Verification items for the finished model (mm, model axes). A direction names the side the tool comes from. Give positions to 0.01 mm unless a question says otherwise; leave off trailing zeros. Order: outer loops, then holes, each group sorted by start corner. A loop starts at its lowest first (then second) coordinate and runs counter-clockwise, first axis right, second up.
(1) Scan lines: L1, parallel to X at y = 32, z = 26.7; L2, parallel to Y at x = 66.5, z = 3.4; L3, parallel to X at y = -24, z = 17.5. Record each from-to range of solid material in increasing order.
(2) Sectioned sample at B-B on y = 4. Record the cut outline in (x, z), plus the area to 3 significant figures.
(3) Gauge pin test, flat ends, axial feed: pin 1 (2.5 mm diameter, centred on y = -32.5, z = 28, fed in from +X); pin 2 (1.5 mm diameter, centred on y = -30.5, z = 1, fed in from -X); pin 3 (12 mm diameter, centred on x = 47, z = 1, fed in from -Y); pin 4 (1.5 mm diameter, centred on x = 37.5, y = -25, fed in from +Z). Record the tip position at first contact, or that the pin passes through.
(4) Sectioned sample at A-A on x = -55.5. Record the cut outline in (y, z), plus the area to 3 significant figures.
(5) Access from +Z, -Z, +X, -X, +Y, -Y to the whole of each face (thin tool, end or side, straight path). Record for faces 1 (the face through (59.5, 32, 28)), 2 (the face through (69.5, 32, 28)), 3 (the face through (-59.5, -32, -3)).
(6) Mould release check, pull along Y, two halves, no side actions. Record for faces 4 (the face through (-69.5, -32, 28)), 5 (the face through (66.24, -20.517, 2.465)), 6 (the face through (60.93, 38, -2.97)), 7 (the face through (-68.07, -38, -2.97)): pulls with the +Y half, pulls with the -Y half, needs draft (parallel to the pull), parting line crosses it, or undercut.
```python
from build123d import *

# Parameters (mm, degrees)
F0_W      = 149
F0_H      = 59
F0_W_2    = 145
F0_H_2    = 55
F1_DEPTH  = 30
F2_W      = 149
F2_H      = 59
F2_W_2    = 145
F2_H_2    = 55
F3_DEPTH  = 5
F4_R      = 2
F4_R_2    = 0.75
F5_DEPTH  = 5
F6_W      = 10
F6_H      = 10
F6_R      = 2.125
F7_DEPTH  = 4
F8_R      = 4.99999
F9_W      = 32.75
F9_H      = 10
F9_W_2    = 30
F10_DEPTH = 2
F11_W     = 10
F11_H     = 5
F12_DEPTH = 5
F14_DEPTH = 144.001
F16_D     = 2
F16_DEPTH = 5
F16_TIP   = 0.600860619


# Not quite as in the source:
# - a fillet or chamfer is up to 0.001 mm smaller than in the source, because OpenCascade refuses the exact size


with BuildPart() as f1:
    # F0 (on Top) → F1 (new body)
    with BuildSketch(Plane.XY):
        Rectangle(F0_W, F0_H)
        Rectangle(F0_W_2, F0_H_2, mode=Mode.SUBTRACT)
    extrude(amount=F1_DEPTH)

    # F2 (on face) → F3 (join)
    with BuildSketch(Plane(origin=(0, 0, 0), x_dir=(1, 0, 0), z_dir=(0, 0, -1))):
        Rectangle(F2_W, F2_H)
        Rectangle(F2_W_2, F2_H_2, mode=Mode.SUBTRACT)
        Rectangle(F2_W_2, F2_H_2)
    extrude(amount=F3_DEPTH)

    # F4 (on face) → F5 (join)
    with BuildSketch(Plane.XY):
        with Locations((-66.5, 22.5)):
            Circle(F4_R)
        with Locations((-66.5, 22.5)):
            Circle(F4_R_2, mode=Mode.SUBTRACT)
        with Locations((-66.5, -22.5)):
            Circle(F4_R)
        with Locations((-66.5, -22.5)):
            Circle(F4_R_2, mode=Mode.SUBTRACT)
        with Locations((66.5, -22.5)):
            Circle(F4_R)
        with Locations((66.5, -22.5)):
            Circle(F4_R_2, mode=Mode.SUBTRACT)
        with Locations((66.5, 22.5)):
            Circle(F4_R)
        with Locations((66.5, 22.5)):
            Circle(F4_R_2, mode=Mode.SUBTRACT)
    extrude(amount=F5_DEPTH)

    # F6 (on face) → F7 (join)
    with BuildSketch(Plane(origin=(0, 0, -5), x_dir=(1, 0, 0), z_dir=(0, 0, -1))):
        with Locations((-64.5, 34.5)):
            Rectangle(F6_W, F6_H)
        with Locations((-64.5, 34.5)):
            Circle(F6_R, mode=Mode.SUBTRACT)
        with Locations((64.5, 34.5)):
            Rectangle(F6_W, F6_H)
        with Locations((64.5, 34.5)):
            Circle(F6_R, mode=Mode.SUBTRACT)
        with Locations((-64.5, -34.5)):
            Rectangle(F6_W, F6_H)
        with Locations((-64.5, -34.5)):
            Circle(F6_R, mode=Mode.SUBTRACT)
        with Locations((64.5, -34.5)):
            Rectangle(F6_W, F6_H)
        with Locations((64.5, -34.5)):
            Circle(F6_R, mode=Mode.SUBTRACT)
    extrude(amount=-F7_DEPTH)

    # F8 (radius 5 in the source; OpenCascade refuses exactly that, so slightly less here)
    f8_edges = [f1.edges().sort_by_distance(p)[0] for p in [
        (-69.5, -39.5, -3),
        (-59.5, -39.5, -3),
        (69.5, -39.5, -3),
        (59.5, -39.5, -3),
        (69.5, 39.5, -3),
        (59.5, 39.5, -3),
        (-59.5, 39.5, -3),
        (-69.5, 39.5, -3),
    ]]
    fillet(f8_edges, radius=F8_R)

    # F9 (on face) → F10 (cut, through all)
    with BuildSketch(Plane(origin=(0, 29.5, 0), x_dir=(-1, 0, 0), z_dir=(0, 1, 0))):
        with Locations((-48.625, 11)):
            Rectangle(F9_W, F9_H)
        with Locations((-15.75, 11)):
            Rectangle(F9_W_2, F9_H)
        with Locations((15.75, 11)):
            Rectangle(F9_W_2, F9_H)
        with Locations((48.625, 11)):
            Rectangle(F9_W, F9_H)
    extrude(amount=-F10_DEPTH, mode=Mode.SUBTRACT)

    # F11 (on face) → F12 (join)
    with BuildSketch(Plane.XY.offset(30)):
        with Locations((64.5, 32)):
            Rectangle(F11_W, F11_H)
        with Locations((-64.5, 32)):
            Rectangle(F11_W, F11_H)
        with Locations((-64.5, -32)):
            Rectangle(F11_W, F11_H)
        with Locations((64.5, -32)):
            Rectangle(F11_W, F11_H)
    extrude(amount=-F12_DEPTH)

    # F13 (on face) → F14 (cut, through all)
    with BuildSketch(Plane(origin=(-69.5, 0, 0), x_dir=(0, -1, 0), z_dir=(-1, 0, 0))):
        Polygon((34.5, 27), (29.5, 25), (34.5, 25), align=None)
        Polygon((-29.5, 25), (-34.5, 27), (-34.5, 25), align=None)
    extrude(amount=-F14_DEPTH, mode=Mode.SUBTRACT)

    # F16
    with Locations(Plane.XY.offset(30)):
        with Locations((64.5, 32), (64.5, -32), (-64.5, -32), (-64.5, 32)):
            Hole(F16_D / 2, depth=F16_DEPTH)
            with Locations((0, 0, -(F16_DEPTH + F16_TIP / 2))):  # 118° drill point
                Cone(0, F16_D / 2, F16_TIP, mode=Mode.SUBTRACT)


solid = f1.part
```
Ans:
1. L1: x = -69.5 to -65.5, -63.5 to -59.5, 59.5 to 63.5, 65.5 to 69.5
1. L2: y = -29.5 to -27.5, -24.5 to -23.25, -21.75 to -20.5, 20.5 to 21.75, 23.25 to 24.5, 27.5 to 29.5
1. L3: x = -74.5 to -72.5, 72.5 to 74.5
2. outline: (-74.5, -5) - (74.5, -5) - (74.5, 30) - (72.5, 30) - (72.5, 0) - (-72.5, 0) - (-72.5, 30) - (-74.5, 30) - close
2. area: 865 mm2
3. pin 1: stops at x = 69.5
3. pin 2: passes through
3. pin 3: stops at y = -29.5
3. pin 4: stops at z = 0
4. outline: (-29.5, -5) - (29.5, -5) - (29.5, 6) - (27.5, 6) - (27.5, 0) - (-27.5, 0) - (-27.5, 30) - (-29.5, 30) - close; (27.5, 16) - (29.5, 16) - (29.5, 30) - (27.5, 30) - close
4. area: 395 mm2
5. face 1: +Z, -Z, +Y
5. face 2: +Z, -Z, +X, +Y
5. face 3: +Z, -Z, -Y
6. face 4: needs draft
6. face 5: undercut
6. face 6: pulls with the +Y half
6. face 7: pulls with the -Y half
